from build123d import *

# Parameters (mm, degrees)
F1_DEPTH = 9
F2_W     = 2
F2_H     = 4.25
F3_DEPTH = 18.3796796564


# Not quite as in the source:
# - a feature names something its author has since deleted; it is built from what else it names


with BuildPart() as f1:
    # F0 (on Front) → F1 (new body)
    with BuildSketch(Plane.XZ):
        with BuildLine():
            Line((-9, -4.5), (9, -4.5))
            Line((9, -4.5), (11, -4.5))
            Line((11, -4.5), (11, -4))
            Line((11, -4), (9, -4))
            Line((9, -4), (9, 4.5))
            Line((9, 4.5), (9, 10))
            Line((9, 10), (5.5606601718, 13.4393398282))
            ThreePointArc((5.5606601718, 13.4393398282), (4.5, 13.8786796564), (3.4393398282, 13.4393398282))
            Line((3.4393398282, 13.4393398282), (0, 10))
            Line((0, 10), (0, 4.5))
            Line((0, 4.5), (-9, 4.5))
            Line((-9, 4.5), (-9, -4.5))
        make_face()
        with BuildLine():
            Line((11, -4), (11, -4.5))
            Line((11, -4.5), (29, -4.5))
            Line((29, -4.5), (31, -4.5))
            Line((31, -4.5), (31, -4))
            Line((31, -4), (29, -4))
            Line((29, -4), (29, 4.5))
            Line((29, 4.5), (29, 10))
            Line((29, 10), (25.5606601718, 13.4393398282))
            ThreePointArc((25.5606601718, 13.4393398282), (24.5, 13.8786796564), (23.4393398282, 13.4393398282))
            Line((23.4393398282, 13.4393398282), (20, 10))
            Line((20, 10), (20, 4.5))
            Line((20, 4.5), (11, 4.5))
            Line((11, 4.5), (11, -4))
        make_face()
        with BuildLine():
            Line((31, -4), (31, -4.5))
            Line((31, -4.5), (49, -4.5))
            Line((49, -4.5), (51, -4.5))
            Line((51, -4.5), (51, -4))
            Line((51, -4), (49, -4))
            Line((49, -4), (49, 4.5))
            Line((49, 4.5), (49, 10))
            Line((49, 10), (45.5606601718, 13.4393398282))
            ThreePointArc((45.5606601718, 13.4393398282), (44.5, 13.8786796564), (43.4393398282, 13.4393398282))
            Line((43.4393398282, 13.4393398282), (40, 10))
            Line((40, 10), (40, 4.5))
            Line((40, 4.5), (31, 4.5))
            Line((31, 4.5), (31, -4))
        make_face()
        with BuildLine():
            Line((51, -4), (51, -4.5))
            Line((51, -4.5), (69, -4.5))
            Line((69, -4.5), (71, -4.5))
            Line((71, -4.5), (71, -4))
            Line((71, -4), (69, -4))
            Line((69, -4), (69, 4.5))
            Line((69, 4.5), (69, 10))
            Line((69, 10), (65.5606601718, 13.4393398282))
            ThreePointArc((65.5606601718, 13.4393398282), (64.5, 13.8786796564), (63.4393398282, 13.4393398282))
            Line((63.4393398282, 13.4393398282), (60, 10))
            Line((60, 10), (60, 4.5))
            Line((60, 4.5), (51, 4.5))
            Line((51, 4.5), (51, -4))
        make_face()
    extrude(amount=-F1_DEPTH)

    # F2 (on face) → F3 (cut, through all)
    with BuildSketch(Plane(origin=(0, 0, -4.5), x_dir=(1, 0, 0), z_dir=(0, 0, -1))):
        with Locations((10, -2.125)):
            Rectangle(F2_W, F2_H)
        with Locations((10, -6.875)):
            Rectangle(F2_W, F2_H)
        with Locations((30, -2.125)):
            Rectangle(F2_W, F2_H)
        with Locations((30, -6.875)):
            Rectangle(F2_W, F2_H)
        with Locations((50, -2.125)):
            Rectangle(F2_W, F2_H)
        with Locations((50, -6.875)):
            Rectangle(F2_W, F2_H)
        with Locations((70, -2.125)):
            Rectangle(F2_W, F2_H)
        with Locations((70, -6.875)):
            Rectangle(F2_W, F2_H)
    extrude(amount=-F3_DEPTH, mode=Mode.SUBTRACT)


solid = f1.part
CAD build for the part. Positions are in the model's coordinates, mm. A direction names the side the tool comes from. Coordinates: 2 decimals unless noted, no trailing zeros. Write each loop counter-clockwise with the first axis right and the second up, starting at its lowest first coordinate (ties: lowest second). Pieces come first, ordered by that corner, then holes. Notation, with made-up numbers: (14.25, 25.5) - (47.25, 25.5) arc R29 cw to (47.25, 53.5) - close; hole circle Ø11 at (42, 1). An arc over 180 degrees is marked (long way). Use a Markdown table: item, result. Add a question column.
Item 1: Band-saw the part on B-B, the plane y = 1.25. Give the number of separate pieces and of enclosed holes in the cut face, and give its area (3 significant figures).
Item 2: Flat gauge pins, fed straight in: pin 1 (4.5 mm diameter, centred on y = 4.5, z = 7, fed in from -X); pin 2 (5 mm diameter, centred on y = 1.5, z = 0, fed in from +X); pin 3 (2.5 mm diameter, centred on x = 57.5, y = 3, fed in from +Z). Where does each tip first touch, or does it go through?
Item 3: Drill centre lines: L1, parallel to X at y = 3, z = 7.5; L2, parallel to X at y = 6.5, z = -1.75; L3, parallel to Z at x = 38, y = 5.5. Where is each one in solid material? Low to high. Write a range as from..to.
Item 4: Band-saw the part on A-A, the plane z = 11. Give the cut face in (x, y).
Item 5: 3-axis set-ups, long thin cutter, end or side, ignore diameter. For faces 4 (the face through (47, 4, 12)), 5 (the face through (62, 9, 3)), 6 (the face through (-4, 4, 4.5)): which of +Z, -Z, +X, -X, +Y, -Y reach the whole face in a straight line?
Item 6: Band-saw the part on D-D, the plane x = 37.5. Give the cut face in (y, z), and give its area (3 significant figures).
Item 7: Mould opens along X. For faces 1 (the face through (42, 4, 12)), 2 (the face through (62, 0, 3)), 3 (the face through (2, 4, 12)) say: pulls with the +X half, pulls with the -X half, needs draft (parallel to the pull), parting line crosses it, or undercut.
Item 8: Band-saw the part on C-C, the plane z = 2.75. Give the cut face in (x, y), and give its area (3 significant figures).
Numbers:
| question | item | result |
|---|---|---|
| 1 | separate pieces | 4 |
| 1 | enclosed holes | 0 |
| 1 | area | 925 mm2 |
| 2 | pin 1 | x = 0 |
| 2 | pin 2 | x = 69 |
| 2 | pin 3 | z = 4.5 |
| 3 | L1 | 0..9, 20..29, 40..49, 60..69 |
| 3 | L2 | -9..9, 11..29, 31..49, 51..69 |
| 3 | L3 | -4.5..4.5 |
| 4 | outline | (1, 0) - (8, 0) - (8, 9) - (1, 9) - close; (21, 0) - (28, 0) - (28, 9) - (21, 9) - close; (41, 0) - (48, 0) - (48, 9) - (41, 9) - close; (61, 0) - (68, 0) - (68, 9) - (61, 9) - close |
| 5 | face 4 | +Z, +Y, -Y |
| 5 | face 5 | +Z, -Z, +X, -X, +Y |
| 5 | face 6 | +Z, -X, +Y, -Y |
| 6 | outline | (0, -4.5) - (9, -4.5) - (9, 4.5) - (0, 4.5) - close |
| 6 | area | 81.0 mm2 |
| 7 | face 1 | undercut |
| 7 | face 2 | needs draft |
| 7 | face 3 | pulls with the -X half |
| 8 | outline | (-9, 0) - (9, 0) - (9, 9) - (-9, 9) - close; (11, 0) - (29, 0) - (29, 9) - (11, 9) - close; (31, 0) - (49, 0) - (49, 9) - (31, 9) - close; (51, 0) - (69, 0) - (69, 9) - (51, 9) - close |
| 8 | area | 648 mm2 |
